Part print with two shaded views. Sizes in mm from the minimum x, y, z corner. A direction names the side the tool comes from. Round coordinates to 2 decimals unless told otherwise and drop trailing zeros. Loops run counter-clockwise (first coordinate to the right, second up) from the corner with the lowest first, then second, coordinate; pieces in that order, holes last. Notation, with made-up numbers: (-11.5, 7.5) -> (16.5, 7.5) arc R30 ccw to (16.5, 30.5) -> close; hole circle Ø10 at (-33, 69.25). An arc over 180 degrees is marked (long way). Answer as a JSON object with one key per item and string values. Group by question number.
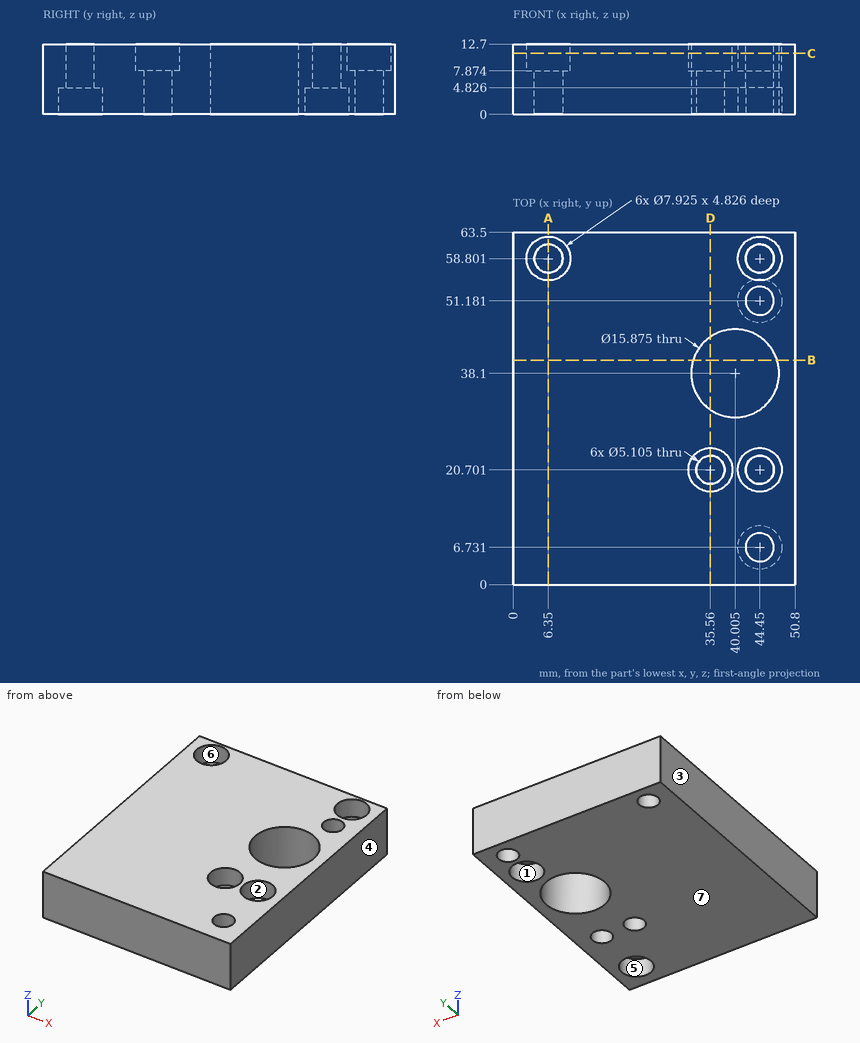
Item 1: Drill centre lines: line 1 (X direction, y = 59, z = 6) (1 decimal); line 2 (Y direction, x = 44.45, z = 10.75) (1 decimal); line 3 (Y direction, x = 44, z = 12.25) (1 decimal). Where is each one in solid material? Low to high.
Item 2: Which spindle directions (+Z, -Z, +X, -X, +Y, -Y) get a long thin tool onto all of the face, cutting with end or side? Do the marked faces 1, 2 and 3. Say none if no direction does.
Item 3: Band-saw the part on A-A, the plane x = 6.35. List the corners of the cut face in (y, z).
Item 4: Two-plate mould, pull along X, no slides. Class the marked faces 4, 5, 6 and 7: pulls with the +X half, pulls with the -X half, needs draft (parallel to the pull), parting line crosses it, or undercut.
Item 5: Band-saw the part on D-D, the plane x = 35.56. List the corners of the cut face in (y, z).
Item 6: Band-saw the part on C-C, the plane z = 11. Count the separate pieces of the cut face and the enclosed holes in it, plus the area to 3 significant figures.
Item 7: Band-saw the part on B-B, the plane y = 40.5. List the corners of the cut face in (x, z), plus the area to 3 significant figures.
Item 8: Drop flat-ended pins along their axis: pin 1 Ø1 at (x, z) = (31.5, 6.5) entering from -Y; pin 2 Ø2.5 at (x, y) = (8, 59) entering from +Z. Give the stop position or say it passes through.
Entries:
{
 "1": {"line 1": "0 to 3.8, 8.9 to 41.9, 47 to 50.8", "line 2": "0 to 4.2, 9.3 to 16.7, 24.7 to 31.5, 44.7 to 48.6, 53.7 to 54.8, 62.8 to 63.5", "line 3": "0 to 4.2, 9.2 to 16.8, 24.6 to 31.2, 45 to 48.7, 53.7 to 54.9, 62.7 to 63.5"},
 "2": {"face 1": "-Z", "face 2": "+Z", "face 3": "+Z, -Z, -X, +Y, -Y"},
 "3": {"outline": "(0, 0) -> (56.25, 0) -> (56.25, 7.87) -> (54.84, 7.87) -> (54.84, 12.7) -> (0, 12.7) -> close; (61.35, 0) -> (63.5, 0) -> (63.5, 12.7) -> (62.76, 12.7) -> (62.76, 7.87) -> (61.35, 7.87) -> close"},
 "4": {"face 4": "pulls with the +X half", "face 5": "undercut", "face 6": "undercut", "face 7": "needs draft"},
 "5": {"outline": "(0, 0) -> (18.15, 0) -> (18.15, 7.87) -> (16.74, 7.87) -> (16.74, 12.7) -> (0, 12.7) -> close; (23.25, 0) -> (31.52, 0) -> (31.52, 12.7) -> (24.66, 12.7) -> (24.66, 7.87) -> (23.25, 7.87) -> close; (44.68, 0) -> (63.5, 0) -> (63.5, 12.7) -> (44.68, 12.7) -> close"},
 "6": {"separate pieces": "1", "enclosed holes": "7", "area": "2,790 mm²"},
 "7": {"outline": "(0, 0) -> (32.44, 0) -> (32.44, 12.7) -> (0, 12.7) -> close; (47.57, 0) -> (50.8, 0) -> (50.8, 12.7) -> (47.57, 12.7) -> close", "area": "453 mm²"},
 "8": {"pin 1": "y = 0", "pin 2": "z = 7.87"}
}
